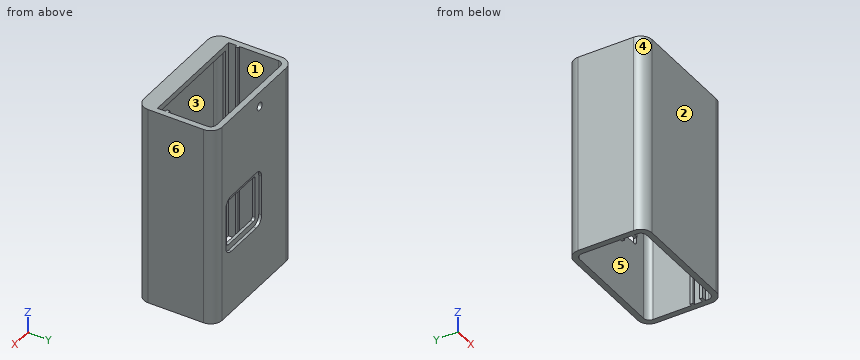
```python
from build123d import *

# Parameters (mm, degrees)
BOSS_EXTRUDE1_DEPTH                 = 88.9
SKETCH2_W                           = 50.419
SKETCH2_H                           = 2.54
BOSS_EXTRUDE2_DEPTH                 = 6.223
F_3_0MM_CLEARANCE_DOWEL_HOLE1_D     = 3.5
F_3_0MM_CLEARANCE_DOWEL_HOLE1_DEPTH = 2.54
CUT_EXTRUDE1_DEPTH                  = 7.62
CUT_EXTRUDE2_DEPTH                  = 1.27


with BuildPart() as part:
    # Sketch1 → Boss-Extrude1 (new body)
    with BuildSketch(Plane.XY):
        with BuildLine():
            Line((17.122726154, 10.071647692), (17.122726154, 34.626647692))
            ThreePointArc((17.122726154, 34.626647692), (15.634828602, 38.218750141), (12.042726154, 39.706647692))
            Line((12.042726154, 39.706647692), (-33.296273846, 39.706647692))
            ThreePointArc((-33.296273846, 39.706647692), (-36.888376295, 38.218750141), (-38.376273846, 34.626647692))
            Line((-38.376273846, 34.626647692), (-38.376273846, 10.071647692))
            ThreePointArc((-38.376273846, 10.071647692), (-36.888376295, 6.479545244), (-33.296273846, 4.991647692))
            Line((-33.296273846, 4.991647692), (12.042726154, 4.991647692))
            ThreePointArc((12.042726154, 4.991647692), (15.634828602, 6.479545244), (17.122726154, 10.071647692))
        make_face()
        with BuildLine():
            Line((-35.836273846, 16.211647692), (-34.820273846, 16.211647692))
            Line((-34.820273846, 16.211647692), (-34.820273846, 17.481647692))
            Line((-34.820273846, 17.481647692), (-35.836273846, 17.481647692))
            Line((-35.836273846, 17.481647692), (-35.836273846, 34.626647692))
            ThreePointArc((-35.836273846, 34.626647692), (-35.09232507, 36.422698917), (-33.296273846, 37.166647692))
            Line((-33.296273846, 37.166647692), (12.042726154, 37.166647692))
            ThreePointArc((12.042726154, 37.166647692), (13.838777378, 36.422698917), (14.582726154, 34.626647692))
            Line((14.582726154, 34.626647692), (14.582726154, 17.481647692))
            Line((14.582726154, 17.481647692), (13.566726154, 17.481647692))
            Line((13.566726154, 17.481647692), (13.566726154, 16.211647692))
            Line((13.566726154, 16.211647692), (14.582726154, 16.211647692))
            Line((14.582726154, 16.211647692), (14.582726154, 12.611647692))
            Line((14.582726154, 12.611647692), (12.550726154, 12.611647692))
            Line((12.550726154, 12.611647692), (12.550726154, 11.341647692))
            Line((12.550726154, 11.341647692), (14.582726154, 11.341647692))
            Line((14.582726154, 11.341647692), (14.582726154, 10.071647692))
            ThreePointArc((14.582726154, 10.071647692), (13.838777378, 8.275596468), (12.042726154, 7.531647692))
            Line((12.042726154, 7.531647692), (-33.296273846, 7.531647692))
            ThreePointArc((-33.296273846, 7.531647692), (-35.09232507, 8.275596468), (-35.836273846, 10.071647692))
            Line((-35.836273846, 10.071647692), (-35.836273846, 11.341647692))
            Line((-35.836273846, 11.341647692), (-33.804273846, 11.341647692))
            Line((-33.804273846, 11.341647692), (-33.804273846, 12.611647692))
            Line((-33.804273846, 12.611647692), (-35.836273846, 12.611647692))
            Line((-35.836273846, 12.611647692), (-35.836273846, 16.211647692))
        make_face(mode=Mode.SUBTRACT)
    extrude(amount=BOSS_EXTRUDE1_DEPTH)

    # Sketch2 → Boss-Extrude2 (add)
    with BuildSketch(Plane(origin=(0, 12.611647692, 0), x_dir=(1, 0, 0), z_dir=(0, 1, 0))):
        with Locations((-10.626773846, -87.63)):
            Rectangle(SKETCH2_W, SKETCH2_H)
    extrude(amount=-BOSS_EXTRUDE2_DEPTH)

    # Ø3.0mm Clearance Dowel Hole1
    with Locations(Plane(origin=(-44.550497372, 37.166647692, -20.932340184), x_dir=(-1, 0, 0), z_dir=(0, -1, 0))):
        with Locations((-30.050223526, -103.406140184)):
            Hole(F_3_0MM_CLEARANCE_DOWEL_HOLE1_D / 2, depth=F_3_0MM_CLEARANCE_DOWEL_HOLE1_DEPTH)

    # Sketch7 → Cut-Extrude1 (cut)
    with BuildSketch(Plane(origin=(0, 39.706647692, 0), x_dir=(1, 0, 0), z_dir=(0, 1, 0))):
        with BuildLine():
            Line((6.962726154, -31.75), (6.962726154, -49.53))
            ThreePointArc((6.962726154, -49.53), (6.590751766, -50.428025612), (5.692726154, -50.8))
            Line((5.692726154, -50.8), (-12.087273846, -50.8))
            ThreePointArc((-12.087273846, -50.8), (-12.985299458, -50.428025612), (-13.357273846, -49.53))
            Line((-13.357273846, -49.53), (-13.357273846, -31.75))
            ThreePointArc((-13.357273846, -31.75), (-12.985299458, -30.851974388), (-12.087273846, -30.48))
            Line((-12.087273846, -30.48), (5.692726154, -30.48))
            ThreePointArc((5.692726154, -30.48), (6.590751766, -30.851974388), (6.962726154, -31.75))
        make_face()
    extrude(amount=-CUT_EXTRUDE1_DEPTH, mode=Mode.SUBTRACT)

    # Sketch7<3> → Cut-Extrude2 (cut)
    with BuildSketch(Plane(origin=(0, 39.706647692, 0), x_dir=(1, 0, 0), z_dir=(0, 1, 0))):
        with BuildLine():
            Line((5.692726154, -27.94), (-12.087273846, -27.94))
            ThreePointArc((-12.087273846, -27.94), (-14.781350682, -29.055923164), (-15.897273846, -31.75))
            Line((-15.897273846, -31.75), (-15.897273846, -49.53))
            ThreePointArc((-15.897273846, -49.53), (-14.781350682, -52.224076836), (-12.087273846, -53.34))
            Line((-12.087273846, -53.34), (5.692726154, -53.34))
            ThreePointArc((5.692726154, -53.34), (8.38680299, -52.224076836), (9.502726154, -49.53))
            Line((9.502726154, -49.53), (9.502726154, -31.75))
            ThreePointArc((9.502726154, -31.75), (8.38680299, -29.055923164), (5.692726154, -27.94))
        make_face()
        with BuildLine():
            Line((6.962726154, -31.75), (6.962726154, -49.53))
            ThreePointArc((6.962726154, -49.53), (6.590751766, -50.428025612), (5.692726154, -50.8))
            Line((5.692726154, -50.8), (-12.087273846, -50.8))
            ThreePointArc((-12.087273846, -50.8), (-12.985299458, -50.428025612), (-13.357273846, -49.53))
            Line((-13.357273846, -49.53), (-13.357273846, -31.75))
            ThreePointArc((-13.357273846, -31.75), (-12.985299458, -30.851974388), (-12.087273846, -30.48))
            Line((-12.087273846, -30.48), (5.692726154, -30.48))
            ThreePointArc((5.692726154, -30.48), (6.590751766, -30.851974388), (6.962726154, -31.75))
        make_face(mode=Mode.SUBTRACT)
    extrude(amount=-CUT_EXTRUDE2_DEPTH, mode=Mode.SUBTRACT)


solid = part.part
```
Read the model definition and answer for the solid it produces. Units are mm, in the model's axes. Face numbers are marked on the shaded views. A direction names the side the tool comes from. Give positions to 0.01 mm unless a question says otherwise; leave off trailing zeros. Order: outer loops, then holes, each group sorted by start corner. A loop starts at its lowest first (then second) coordinate and runs counter-clockwise, first axis right, second up.
(1) Find section A-A (y = 31). Give the vertices of the cut face in (x, z).
(2) Given pin 1 (0.8 mm diameter, centred on x = -35.5, z = 39.5, fed in from +Y); pin 2 (1.6 mm diameter, centred on x = -35, z = 28.5, fed in from -Y); pin 3 (3 mm diameter, centred on x = -14.5, z = 82.47, fed in from +Y), each flat-ended and moving along its own axis, determine where each tip first touches the part or whether it passes through.
(3) Find section C-C (x = -27). Give the vertices of the cut face in (y, z), plus the area to 3 significant figures.
(4) For a pull along X with two mould halves and no side action, classify the marked faces 1, 2, 3 and 4 as released by +X, released by -X, zero draft, split by the parting line, or undercut.
(5) For the marked faces 5 and 6, determine the directions among +Z, -Z, +X, -X, +Y, -Y from which every point of the face is accessible in a straight line to the end or side of a thin tool.
(6) Straight lines are drawn through the part: L1, parallel to Y at x = -24, z = 44; L2, parallel to X at y = 32.5, z = 57; L3, parallel to X at y = 16.5, z = 83. For each, find the intervals that lie inside material, in ascending order.
Result sheet:
1. outline: (-38.38, 0) - (-35.84, 0) - (-35.84, 88.9) - (-38.38, 88.9) - close; (14.58, 0) - (17.12, 0) - (17.12, 88.9) - (14.58, 88.9) - close
2. pin 1: stops at y = 39.38
2. pin 2: stops at y = 5.07
2. pin 3: stops at y = 7.53
3. outline: (4.99, 0) - (7.53, 0) - (7.53, 86.36) - (12.61, 86.36) - (12.61, 88.9) - (4.99, 88.9) - close; (37.17, 0) - (39.71, 0) - (39.71, 88.9) - (37.17, 88.9) - close
3. area: 465 mm2
4. face 1: undercut
4. face 2: zero draft
4. face 3: undercut
4. face 4: released by -X
5. face 5: +Z, -Z
5. face 6: +Z, -Z, +X, +Y, -Y
6. L1: y = 4.99 to 7.53, 37.17 to 39.71
6. L2: x = -38.38 to -35.84, 14.58 to 17.12
6. L3: x = -38.38 to -34.82, 13.57 to 17.12
